Geometry check sheet. Reference: the model listing, model coordinates, mm. Face numbers are marked on the shaded views. Round coordinates to 2 decimals unless told otherwise and drop trailing zeros. Loops run counter-clockwise (first coordinate to the right, second up) from the corner with the lowest first, then second, coordinate; pieces in that order, holes last. Notation, with made-up numbers: (56.5, 48.25) - (79.5, 48.25) arc R19 cw to (79.5, 64.25) - close; hole circle Ø11 at (13, 55). An arc over 180 degrees is marked (long way). Write item = value, one per line.
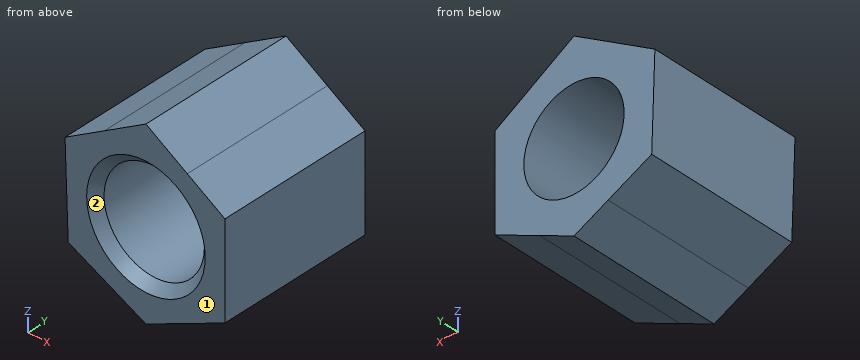
```python
from build123d import *

# Parameters (mm, degrees)
F0_R     = 2.75
F1_DEPTH = 8.45
F2_SIZE  = 0.5


with BuildPart() as f1:
    # F0 (on Front) → F1 (new body)
    with BuildSketch(Plane.XZ):
        with BuildLine():
            ThreePointArc((-132.8375352313, 22.8701725471), (-131.0452779523, 24.467741248), (-130.3796414733, 26.7745442275))
            ThreePointArc((-130.3796414733, 26.7745442275), (-130.9300791601, 28.887316984), (-132.441446887, 30.4629305032))
            ThreePointArc((-132.441446887, 30.4629305032), (-134.7096414781, 31.1045442275), (-136.9778360677, 30.4629304982))
            ThreePointArc((-136.9778360677, 30.4629304982), (-139.0337617379, 26.5489695453), (-136.5817476464, 22.8701725141))
            ThreePointArc((-136.5817476464, 22.8701725141), (-134.7096414351, 22.4445442275), (-132.8375352313, 22.8701725471))
        make_face()
        with Locations((-134.7096414733, 26.7745442275)):
            Circle(F0_R, mode=Mode.SUBTRACT)
        with BuildLine():
            Line((-130.3796414733, 24.0487074352), (-130.3796414733, 26.7745442275))
            ThreePointArc((-130.3796414733, 26.7745442275), (-131.0452779523, 24.467741248), (-132.8375352313, 22.8701725471))
            Line((-132.8375352313, 22.8701725471), (-130.3796414733, 24.0487074352))
        make_face()
        with BuildLine():
            ThreePointArc((-132.441446887, 30.4629305032), (-130.9300791601, 28.887316984), (-130.3796414733, 26.7745442275))
            Line((-130.3796414733, 26.7745442275), (-130.3796414733, 29.1950113514))
            Line((-130.3796414733, 29.1950113514), (-132.441446887, 30.4629305032))
        make_face()
        with BuildLine():
            ThreePointArc((-136.9778360677, 30.4629304982), (-134.7096414781, 31.1045442275), (-132.441446887, 30.4629305032))
            Line((-132.441446887, 30.4629305032), (-134.7096414733, 31.8577698691))
            Line((-134.7096414733, 31.8577698691), (-136.9778360677, 30.4629304982))
        make_face()
        with BuildLine():
            Line((-134.7096414733, 21.9725167744), (-132.8375352313, 22.8701725471))
            ThreePointArc((-132.8375352313, 22.8701725471), (-134.7096414351, 22.4445442275), (-136.5817476464, 22.8701725141))
            Line((-136.5817476464, 22.8701725141), (-134.7096414733, 21.9725167744))
        make_face()
        with BuildLine():
            ThreePointArc((-136.5817476464, 22.8701725141), (-139.0337617379, 26.5489695453), (-136.9778360677, 30.4629304982))
            Line((-136.9778360677, 30.4629304982), (-139.1458009268, 29.1297279821))
            Line((-139.1458009268, 29.1297279821), (-138.971331925, 24.0159537063))
            Line((-138.971331925, 24.0159537063), (-136.5817476464, 22.8701725141))
        make_face()
    extrude(amount=F1_DEPTH)

    # F2
    f2_edges = [f1.edges().sort_by_distance(p)[0] for p in [
        (-137.459641, -8.45, 26.774544),
    ]]
    chamfer(f2_edges, length=F2_SIZE)


solid = f1.part
```
(1) Scan lines: L1, parallel to Z at x = -135.5, y = -2.5; L2, parallel to X at y = -3, z = 24.25; L3, parallel to X at y = -6.5, z = 24.75. Record each from-to range of solid material in increasing order. Write a range as [from, to].
Answers follow:
L1 = [22.35, 24.14], [29.41, 31.37]
L2 = [-138.98, -135.8], [-133.62, -130.38]
L3 = [-139, -136.57], [-132.85, -130.38]
(2) Gauge pin test, flat ends, axial feed: pin 1 (5 mm diameter, centred on x = -134.71, z = 26.77, fed in from +Y); pin 2 (3 mm diameter, centred on x = -135.5, y = -3, fed in from +Z); pin 3 (5 mm diameter, centred on x = -133, z = 24, fed in from +Y). Record the tip position at first contact, or that the pin passes through.
Answers follow:
pin_1 = through
pin_2 = 31.86
pin_3 = 0
(3) Section check A-A (y = -7.25). Enter the section's corners in (x, z), then the cut area to 3 significant figures.
Answers follow:
outline = (-139.15, 29.13) - (-138.97, 24.02) - (-134.71, 21.97) - (-130.38, 24.05) - (-130.38, 29.2) - (-134.71, 31.86) - close; hole circle Ø5.5 at (-134.71, 26.77)
area = 41.4 mm²
(4) Mould release check, pull along Z, two halves, no side actions. Record for the marked faces 1 and 2: pulls with the +Z half, pulls with the -Z half, needs draft (parallel to the pull), parting line crosses it, or undercut.
Answers follow:
face_1 = needs draft
face_2 = undercut
